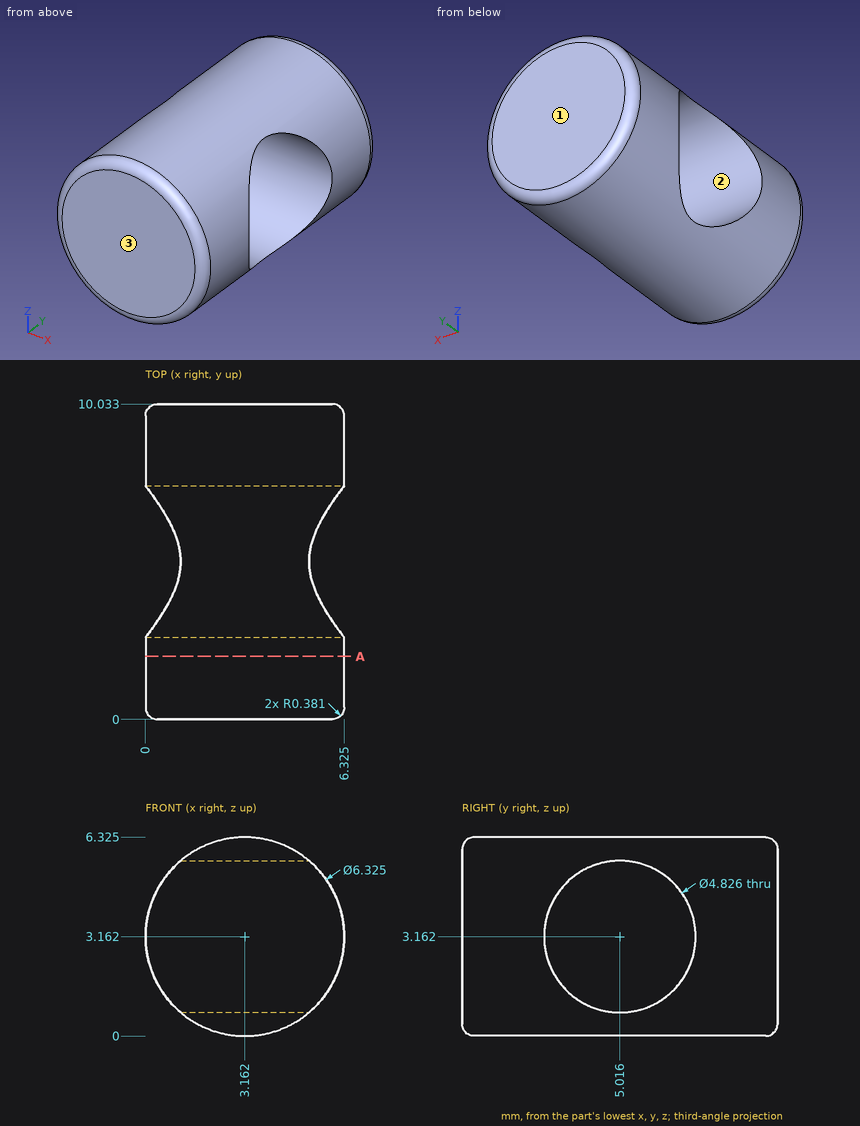
Answer from the drawing. Dimensions are ordinates in mm from the lowest x, y and z of the part. Round coordinates to 2 decimals unless told otherwise and drop trailing zeros. Write each loop counter-clockwise with the first axis right and the second up, starting at its lowest first coordinate (ties: lowest second). Pieces come first, ordered by that corner, then holes.
1. Given pin 1 Ø1 at (x, y) = (3.5, 7) entering from +Z (1 decimal); pin 2 Ø3 at (y, z) = (5.02, 3.16) entering from +X, each flat-ended and moving along its own axis, determine where each tip first touches the part or whether it passes through.
2. Straight lines are drawn through the part: L1, parallel to Y at x = 6, z = 2.75 (1 decimal); L2, parallel to Y at x = 2.5, z = 2 (1 decimal); L3, parallel to Z at x = 5, y = 3 (1 decimal). For each, find the intervals that lie inside material, in ascending order.
3. The part is cut by section A-A, the plane y = 2. Determine the outline of the cut face in (x, z) (1 decimal), then the cut area to 3 significant figures.
4. Determine the mould class of the marked faces 1, 2 and 3 for opening direction Y: pulls with the +Y half, pulls with the -Y half, needs draft (parallel to the pull), parting line crosses it, or undercut.
Values:
1. pin 1: stops at z = 6.3
1. pin 2: passes through
2. L1: y = 0 to 2.6, 7.4 to 10
2. L2: y = 0 to 2.9, 7.1 to 10
2. L3: z = 0.6 to 1.8, 4.5 to 5.7
3. outline: circle Ø6.3 at (3.2, 3.2)
3. area: 31.4 mm2
4. face 1: pulls with the +Y half
4. face 2: undercut
4. face 3: pulls with the -Y half
